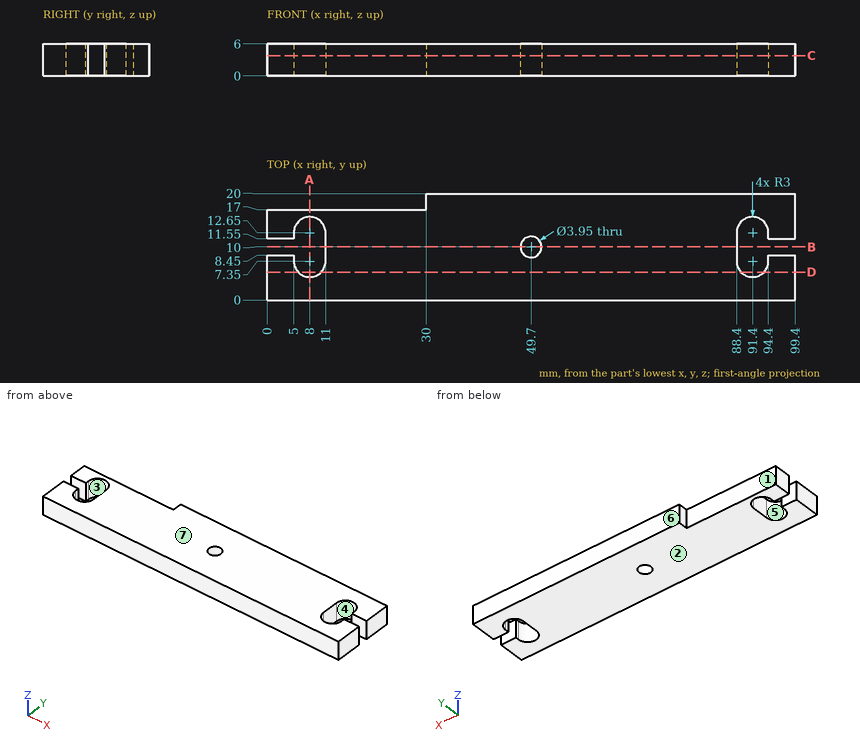
Check sheet for the drawn part. Datum: minimum x, y, z corner. Units: mm. A direction names the side the tool comes from. Give positions to 0.01 mm unless a question says otherwise; leave off trailing zeros. Loops run counter-clockwise (first coordinate to the right, second up) from the corner with the lowest first, then second, coordinate; pieces in that order, holes last.
1) Draft check along Y on the marked faces 4, 5, 6 and 7. Enter one of: pulls with the +Y half, pulls with the -Y half, needs draft (parallel to the pull), parting line crosses it, or undercut.
2) Sectioned sample at D-D, the plane y = 5.25. Enter the section's corners in (x, z).
3) Sectioned sample at A-A, the plane x = 8. Enter the section's corners in (y, z).
4) Sectioned sample at C-C, the plane z = 3.8. Enter the section's corners in (x, y) (3 decimals), then the cut area to 3 significant figures.
5) Sectioned sample at B-B, the plane y = 10. Enter the section's corners in (x, z) (3 decimals).
6) Thickness scan on line 1 along X through (y, z) = (12.5, 4.15); line 2 along Y through (x, z) = (49.7, 1.45) (3 decimals); line 3 along Y through (x, z) = (8, 3.9). Record the ranges inside material, lowest first.
7) Depth check by flat-ended pin: pin 1 Ø1.5 at (y, z) = (19, 4) entering from -X. Enter the tip coordinate at first touch or a pass-through.
8) Set-up check for the marked faces 1, 2 and 3: record each of +Z, -Z, +X, -X, +Y, -Y from which the full face is reachable in a straight line by a thin tool's end or side.
Answers:
1. face 4: undercut
1. face 5: undercut
1. face 6: pulls with the +Y half
1. face 7: needs draft
2. outline: (0, 0) - (5.86, 0) - (5.86, 6) - (0, 6) - close; (10.14, 0) - (89.26, 0) - (89.26, 6) - (10.14, 6) - close; (93.54, 0) - (99.4, 0) - (99.4, 6) - (93.54, 6) - close
3. outline: (0, 0) - (4.35, 0) - (4.35, 6) - (0, 6) - close; (15.65, 0) - (17, 0) - (17, 6) - (15.65, 6) - close
4. outline: (0, 0) - (99.4, 0) - (99.4, 8.45) - (94.4, 8.45) - (94.4, 7.35) arc R3 cw to (88.4, 7.35) - (88.4, 12.65) arc R3 cw to (94.4, 12.65) - (94.4, 11.55) - (99.4, 11.55) - (99.4, 20) - (30, 20) - (30, 17) - (0, 17) - (0, 11.55) - (5, 11.55) - (5, 12.65) arc R3 cw to (11, 12.65) - (11, 7.35) arc R3 cw to (5, 7.35) - (5, 8.45) - (0, 8.45) - close; hole circle Ø3.95 at (49.7, 10)
4. area: 1,730 mm2
5. outline: (11, 0) - (47.725, 0) - (47.725, 6) - (11, 6) - close; (51.675, 0) - (88.4, 0) - (88.4, 6) - (51.675, 6) - close
6. line 1: x = 0 to 5, 11 to 88.4, 94.4 to 99.4
6. line 2: y = 0 to 8.025, 11.975 to 20
6. line 3: y = 0 to 4.35, 15.65 to 17
7. pin 1: stops at x = 30
8. face 1: +Z, -Z, -X, +Y
8. face 2: -Z, +X, -X, +Y, -Y
8. face 3: +Z, -Z
